Read the model definition and answer for the solid it produces. Units are mm, in the model's axes. A direction names the side the tool comes from. Coordinates: 2 decimals unless noted, no trailing zeros. Write each loop counter-clockwise with the first axis right and the second up, starting at its lowest first coordinate (ties: lowest second). Pieces come first, ordered by that corner, then holes. Notation, with made-up numbers: (31, 53) -> (71, 53) arc R10 cw to (71, 69) -> close; hole circle Ø2 at (57.25, 78). An arc over 180 degrees is marked (long way). Use CSV: the item, a comma, the result in double quotes.
from build123d import *

# Parameters (mm, degrees)
SKETCH1_R           = 1.65
SKETCH1_W           = 30.68
SKETCH1_H           = 2.7
BOSS_EXTRUDE1_DEPTH = 2.7


with BuildPart() as part:
    # Sketch1 → Boss-Extrude1 (new body)
    with BuildSketch(Plane(origin=(0, 0, 0), x_dir=(1, 0, 0), z_dir=(0, 1, 0))):
        with BuildLine():
            Line((-46, 0), (46, 0))
            ThreePointArc((46, 0), (62.780941571, 3.32568378), (77.025151087, 12.8))
            Line((77.025151087, 12.8), (46.015151087, 12.8))
            Line((46.015151087, 12.8), (46.015151087, 15.5))
            Line((46.015151087, 15.5), (73.995151087, 15.5))
            Line((73.995151087, 15.5), (73.995151087, 35.5))
            Line((73.995151087, 35.5), (-73.995151087, 35.5))
            Line((-73.995151087, 35.5), (-73.995151087, 15.5))
            Line((-73.995151087, 15.5), (-46.015151087, 15.5))
            Line((-46.015151087, 15.5), (-46.015151087, 12.8))
            Line((-46.015151087, 12.8), (-77.025151087, 12.8))
            ThreePointArc((-77.025151087, 12.8), (-62.780941571, 3.32568378), (-46, 0))
        make_face()
        with Locations((46, 28.5)):
            Circle(SKETCH1_R, mode=Mode.SUBTRACT)
        with Locations((46, 7)):
            Circle(SKETCH1_R, mode=Mode.SUBTRACT)
        with Locations((-46, 7)):
            Circle(SKETCH1_R, mode=Mode.SUBTRACT)
        with Locations((-46, 28.5)):
            Circle(SKETCH1_R, mode=Mode.SUBTRACT)
        with Locations((0, 14.15)):
            Rectangle(SKETCH1_W, SKETCH1_H, mode=Mode.SUBTRACT)
    extrude(amount=BOSS_EXTRUDE1_DEPTH)


solid = part.part
1. A tool of negligible diameter and unlimited length cuts with its end or side. For faces 4 (the flat face through (-46.015, 1, -14)), 5 (the flat face through (-15.34, 1, -14)), 6 (the flat face through (62, 1, -12.8)), from which of +Z, -Z, +X, -X, +Y, -Y can it reach the whole face along a straight path? Write none if from no direction.
Solutions:
face 4,"-X, +Y, -Y"
face 5,"+Y, -Y"
face 6,"+X, +Y, -Y"
2. A cutting plane is placed at B-B (z = -28.5). Give the vertices of the cut face in (x, y).
Solutions:
outline,"(-74, 0) -> (-47.65, 0) -> (-47.65, 2.7) -> (-74, 2.7) -> close; (-44.35, 0) -> (44.35, 0) -> (44.35, 2.7) -> (-44.35, 2.7) -> close; (47.65, 0) -> (74, 0) -> (74, 2.7) -> (47.65, 2.7) -> close"
3. A cutting plane is placed at C-C (y = 1.95). Give the vertices of the cut face in (x, z), and give its area (3 significant figures).
Solutions:
outline,"(-77.03, -12.8) -> (-46.02, -12.8) -> (-46.02, -15.5) -> (-74, -15.5) -> (-74, -35.5) -> (74, -35.5) -> (74, -15.5) -> (46.02, -15.5) -> (46.02, -12.8) -> (77.03, -12.8) arc R44 ccw to (46, 0) -> (-46, 0) arc R44 ccw to start; hole circle Ø3.3 at (-46, -28.5); hole circle Ø3.3 at (-46, -7); hole (-15.34, -15.5) -> (15.34, -15.5) -> (15.34, -12.8) -> (-15.34, -12.8) -> close; hole circle Ø3.3 at (46, -28.5); hole circle Ø3.3 at (46, -7)"
area,"4,820 mm^2"
4. For a pull along X with two mould halves and no side action, classify faces 1 (the flat face through (0, 1, -12.8)), 2 (the cylindrical face through (62.558, 1.331, -3.234)), 3 (the flat face through (-60, 1, -15.5)) as pulls with the +X half, pulls with the -X half, needs draft (parallel to the pull), parting line crosses it, or undercut.
Solutions:
face 1,"undercut"
face 2,"pulls with the +X half"
face 3,"needs draft"
5. A cutting plane is placed at A-A (x = 13). Give the vertices of the cut face in (y, z).
Solutions:
outline,"(0, -35.5) -> (2.7, -35.5) -> (2.7, -15.5) -> (0, -15.5) -> close; (0, -12.8) -> (2.7, -12.8) -> (2.7, 0) -> (0, 0) -> close"
6. A cutting plane is placed at D-D (x = 64). Give the vertices of the cut face in (y, z), and give its area (3 significant figures).
Solutions:
outline,"(0, -35.5) -> (2.7, -35.5) -> (2.7, -15.5) -> (0, -15.5) -> close; (0, -12.8) -> (2.7, -12.8) -> (2.7, -3.85) -> (0, -3.85) -> close"
area,"78.2 mm^2"
7. Each of these flat-tipped pins is pushed along its axis until it touches: pin 1 Ø0.8 at (y, z) = (1.5, -13.5) entering from +X; pin 2 Ø0.8 at (y, z) = (1.5, -14) entering from -X; pin 3 Ø1 at (y, z) = (1.5, -27.5) entering from -X. Where does it stop, or does it pass through?
Solutions:
pin 1,"stops at x = 46.02"
pin 2,"stops at x = -46.02"
pin 3,"stops at x = -74"
8. Find the intervals of material crossed by line 1 along X through (y, z) = (1.05, -28.5); line 2 along X through (y, z) = (1.2, -7.5); line 3 along Z through (x, y) = (0, 0.2), in increasing order.
Solutions:
line 1,"x = -74 to -47.65, -44.35 to 44.35, 47.65 to 74"
line 2,"x = -70.57 to -47.57, -44.43 to 44.43, 47.57 to 70.57"
line 3,"z = -35.5 to -15.5, -12.8 to 0"
